from build123d import *

# Parameters (mm, degrees)
EXTRUDE_1_DEPTH     = 70
FILLET_1_R          = 10
CUT_EXTRUDE_1_REACH = 72
CUT_EXTRUDE_2_REACH = 277
SKETCH_3_R          = 5
EXTRUDE_2_DEPTH     = 3


with BuildPart() as part:
    # 草图1 → 凸台-拉伸1 (new body)
    with BuildSketch(Plane.XY):
        with BuildLine():
            Line((8, 0), (70, 0))
            Line((70, 0), (70, -6))
            Line((70, -6), (8, -6))
            ThreePointArc((8, -6), (6.585786438, -6.585786438), (6, -8))
            Line((6, -8), (6, -275))
            Line((6, -275), (0, -275))
            Line((0, -275), (0, -8))
            ThreePointArc((0, -8), (2.343145751, -2.343145751), (8, 0))
        make_face()
    extrude(amount=EXTRUDE_1_DEPTH)

    # 圆角1
    fillet_1_edges = [part.edges().sort_by_distance(p)[0] for p in [
        (70, -3, 0),
        (3, -275, 70),
        (70, -3, 70),
        (3, -275, 0),
    ]]
    fillet(fillet_1_edges, radius=FILLET_1_R)

    # 草图2 → 切除-拉伸1 (cut, up to next)
    with BuildSketch(Plane.ZY, mode=Mode.PRIVATE) as cut_extrude_1_sk1:
        with BuildLine():
            Line((6.75, -255), (6.75, -265))
            ThreePointArc((6.75, -265), (10, -268.25), (13.25, -265))
            Line((13.25, -265), (13.25, -255))
            ThreePointArc((13.25, -255), (10, -251.75), (6.75, -255))
        make_face()
    cut_extrude_1_tool1 = extrude(cut_extrude_1_sk1.sketch, amount=-CUT_EXTRUDE_1_REACH, mode=Mode.PRIVATE) & part.part
    add(cut_extrude_1_tool1.solids().sort_by_distance((0, -260, 10))[0], mode=Mode.SUBTRACT)
    # 草图2 → 切除-拉伸1 (cut, up to next)
    with BuildSketch(Plane.ZY, mode=Mode.PRIVATE) as cut_extrude_1_sk2:
        with BuildLine():
            Line((22.625, -255), (22.625, -265))
            ThreePointArc((22.625, -265), (25.875, -268.25), (29.125, -265))
            Line((29.125, -265), (29.125, -255))
            ThreePointArc((29.125, -255), (25.875, -251.75), (22.625, -255))
        make_face()
    cut_extrude_1_tool2 = extrude(cut_extrude_1_sk2.sketch, amount=-CUT_EXTRUDE_1_REACH, mode=Mode.PRIVATE) & part.part
    add(cut_extrude_1_tool2.solids().sort_by_distance((0, -260, 25.875))[0], mode=Mode.SUBTRACT)
    # 草图2 → 切除-拉伸1 (cut, up to next)
    with BuildSketch(Plane.ZY, mode=Mode.PRIVATE) as cut_extrude_1_sk3:
        with BuildLine():
            Line((38.5, -255), (38.5, -265))
            ThreePointArc((38.5, -265), (41.75, -268.25), (45, -265))
            Line((45, -265), (45, -255))
            ThreePointArc((45, -255), (41.75, -251.75), (38.5, -255))
        make_face()
    cut_extrude_1_tool3 = extrude(cut_extrude_1_sk3.sketch, amount=-CUT_EXTRUDE_1_REACH, mode=Mode.PRIVATE) & part.part
    add(cut_extrude_1_tool3.solids().sort_by_distance((0, -260, 41.75))[0], mode=Mode.SUBTRACT)
    # 草图2 → 切除-拉伸1 (cut, up to next)
    with BuildSketch(Plane.ZY, mode=Mode.PRIVATE) as cut_extrude_1_sk4:
        with BuildLine():
            Line((54.375, -255), (54.375, -265))
            ThreePointArc((54.375, -265), (57.625, -268.25), (60.875, -265))
            Line((60.875, -265), (60.875, -255))
            ThreePointArc((60.875, -255), (57.625, -251.75), (54.375, -255))
        make_face()
    cut_extrude_1_tool4 = extrude(cut_extrude_1_sk4.sketch, amount=-CUT_EXTRUDE_1_REACH, mode=Mode.PRIVATE) & part.part
    add(cut_extrude_1_tool4.solids().sort_by_distance((0, -260, 57.625))[0], mode=Mode.SUBTRACT)

    # 草图3 → 切除-拉伸2 (cut, up to next)
    with BuildSketch(Plane(origin=(0, 0, 0), x_dir=(1, 0, 0), z_dir=(0, 1, 0)), mode=Mode.PRIVATE) as cut_extrude_2_sk1:
        with Locations((60, -15)):
            Circle(SKETCH_3_R)
    cut_extrude_2_tool1 = extrude(cut_extrude_2_sk1.sketch, amount=-CUT_EXTRUDE_2_REACH, mode=Mode.PRIVATE) & part.part
    add(cut_extrude_2_tool1.solids().sort_by_distance((60, 0, 15))[0], mode=Mode.SUBTRACT)
    # 草图3 → 切除-拉伸2 (cut, up to next)
    with BuildSketch(Plane(origin=(0, 0, 0), x_dir=(1, 0, 0), z_dir=(0, 1, 0)), mode=Mode.PRIVATE) as cut_extrude_2_sk2:
        with Locations((20, -15)):
            Circle(SKETCH_3_R)
    cut_extrude_2_tool2 = extrude(cut_extrude_2_sk2.sketch, amount=-CUT_EXTRUDE_2_REACH, mode=Mode.PRIVATE) & part.part
    add(cut_extrude_2_tool2.solids().sort_by_distance((20, 0, 15))[0], mode=Mode.SUBTRACT)
    # 草图3 → 切除-拉伸2 (cut, up to next)
    with BuildSketch(Plane(origin=(0, 0, 0), x_dir=(1, 0, 0), z_dir=(0, 1, 0)), mode=Mode.PRIVATE) as cut_extrude_2_sk3:
        with Locations((20, -55)):
            Circle(SKETCH_3_R)
    cut_extrude_2_tool3 = extrude(cut_extrude_2_sk3.sketch, amount=-CUT_EXTRUDE_2_REACH, mode=Mode.PRIVATE) & part.part
    add(cut_extrude_2_tool3.solids().sort_by_distance((20, 0, 55))[0], mode=Mode.SUBTRACT)
    # 草图3 → 切除-拉伸2 (cut, up to next)
    with BuildSketch(Plane(origin=(0, 0, 0), x_dir=(1, 0, 0), z_dir=(0, 1, 0)), mode=Mode.PRIVATE) as cut_extrude_2_sk4:
        with Locations((60, -55)):
            Circle(SKETCH_3_R)
    cut_extrude_2_tool4 = extrude(cut_extrude_2_sk4.sketch, amount=-CUT_EXTRUDE_2_REACH, mode=Mode.PRIVATE) & part.part
    add(cut_extrude_2_tool4.solids().sort_by_distance((60, 0, 55))[0], mode=Mode.SUBTRACT)

    # 草图4 → 凸台-拉伸2 (add, symmetric)
    with BuildSketch(Plane(origin=(0, 0, 35), x_dir=(-1, 0, 0), z_dir=(0, 0, -1))):
        Polygon((-6, -14), (-6, -246), (-14, -246), (-66, -14), (-66, -6), (-14, -6), align=None)
    extrude(amount=EXTRUDE_2_DEPTH, both=True)


solid = part.part
Part model, mm, in its own coordinate system. A direction names the side the tool comes from. Give positions to 0.01 mm unless a question says otherwise; leave off trailing zeros. Write each loop counter-clockwise with the first axis right and the second up, starting at its lowest first coordinate (ties: lowest second). Pieces come first, ordered by that corner, then holes.
1) Pin check, flat tips, straight feed: pin 1 (1.5 mm diameter, centred on x = 9.5, y = -95, fed in from -Z); pin 2 (8 mm diameter, centred on x = 60, z = 15, fed in from -Y); pin 3 (1.8 mm diameter, centred on x = 10, z = 35.5, fed in from -Y); pin 4 (16 mm diameter, centred on x = 20, z = 15, fed in from -Y). Stop position of each tip, or through.
Resolved:
pin 1: stops at z = 32
pin 2: passes through
pin 3: stops at y = -246
pin 4: stops at y = -6
2) Two-plate mould, pull along Y, no slides. Class faces 4 (the face through (2.96, -251.75, 41.82)), 5 (the face through (5.7, -102.4, 70)), 6 (the face through (3, -275, 35)): released by +Y, released by -Y, zero draft, split by the parting line, or undercut.
Resolved:
face 4: undercut
face 5: zero draft
face 6: released by -Y
3) Cut at B-B on x = 20. Write the cut outline in (y, z), then the cut area to 3 significant figures.
Resolved:
outline: (-219.23, 32) - (-6, 32) - (-6, 20) - (0, 20) - (0, 50) - (-6, 50) - (-6, 38) - (-219.23, 38) - close; (-6, 0) - (0, 0) - (0, 10) - (-6, 10) - close; (-6, 60) - (0, 60) - (0, 70) - (-6, 70) - close
area: 1,580 mm2
4) Which spindle directions (+Z, -Z, +X, -X, +Y, -Y) get a long thin tool onto all of the face, cutting with end or side? Do faces 1 (the face through (10, -246, 35)), 2 (the face through (19.349, -2.958, 50.043)), 3 (the face through (3, -260, 13.25)). Say none if no direction does.
Resolved:
face 1: +Z, -Z, +X, -Y
face 2: +Y, -Y
face 3: +X, -X
5) Cut at A-A on z = 41.75. Write the cut outline in (x, y).
Resolved:
outline: (0, -275) - (6, -275) - (6, -268.25) - (0, -268.25) - close; (0, -251.75) - (6, -251.75) - (6, -8) arc R2 cw to (8, -6) - (70, -6) - (70, 0) - (8, 0) arc R8 ccw to (0, -8) - close
6) Cut at C-C on y = -178.5. Write the cut outline in (x, z).
Resolved:
outline: (0, 0) - (6, 0) - (6, 32) - (29.13, 32) - (29.13, 38) - (6, 38) - (6, 70) - (0, 70) - close
7) Cut at D-D on z = 25. Write the cut outline in (x, y), then the cut area to 3 significant figures.
Resolved:
outline: (0, -275) - (6, -275) - (6, -268.13) - (0, -268.13) - close; (0, -251.87) - (6, -251.87) - (6, -8) arc R2 cw to (8, -6) - (70, -6) - (70, 0) - (8, 0) arc R8 ccw to (0, -8) - close
area: 1,920 mm2
8) Probe L1, parallel to Z at x = 60, y = -3.9; L2, parallel to X at y = -1, z = 15; L3, parallel to X at y = -2, z = 55. List the from-to ranges inside material, lowest first.
Resolved:
L1: z = 0 to 10, 20 to 50, 60 to 70
L2: x = 4.13 to 15, 25 to 55, 65 to 70
L3: x = 2.71 to 15, 25 to 55, 65 to 70
